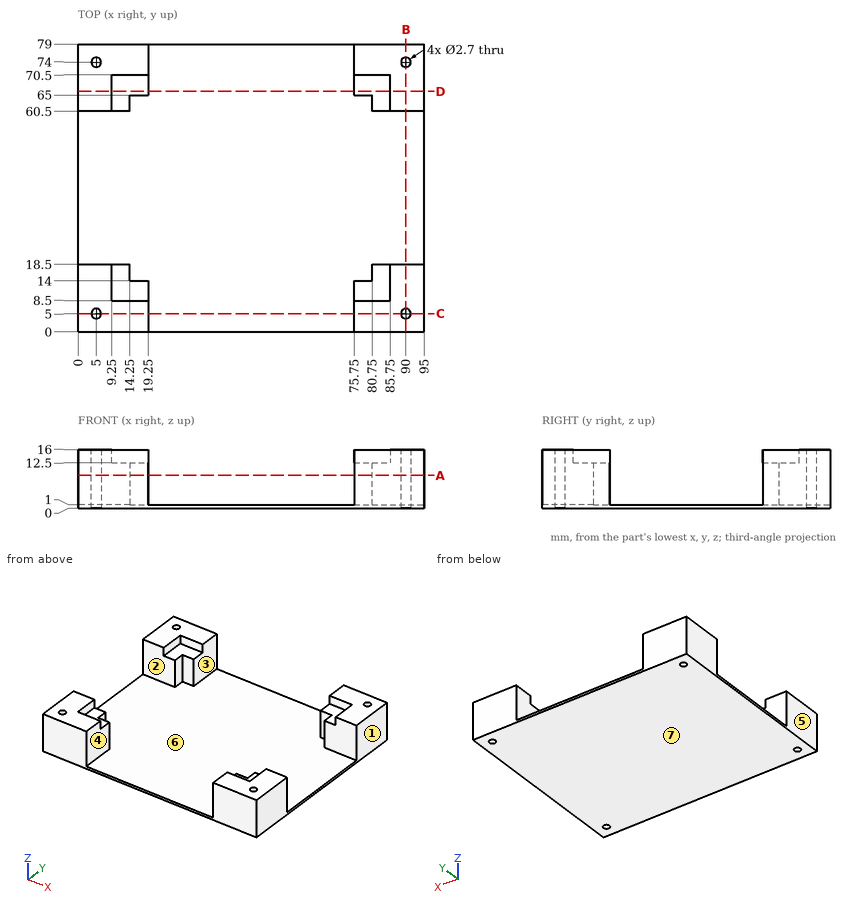
Can you work these out from the drawing? Everything is in mm from the part's minimum corner. A direction names the side the tool comes from. Round coordinates to 2 decimals unless told otherwise and drop trailing zeros. Write each loop counter-clockwise with the first axis right and the second up, starting at its lowest first coordinate (ties: lowest second). Pieces come first, ordered by that corner, then holes.
1. For the marked faces 1, 2 and 3, which set-ups out of +Z, -Z, +X, -X, +Y, -Y let a thin tool reach every point of the face, with its end or its side?
2. If we mould it in two halves opening along X, with no side actions, what happens to the marked faces 4, 5, 6 and 7? For each: released by +X, released by -X, zero draft, split by the parting line, or undercut.
3. I need wall thicknesses on L1, parallel to Y at x = 5, z = 5.25; L2, parallel to X at y = 74, z = 10.5; L3, parallel to Y at x = 79, z = 15.75. Which ranges of each line are inside material? Lowest first, please.
4. Suppose I cut it at D-D (y = 66). List the corners of the cut face in (x, z) for me.
5. Suppose I cut it at C-C (y = 5). List the corners of the cut face in (x, z) for me.
6. Will these pins go through, and if not, where does the flat tip stop? pin 1 Ø12 at (x, y) = (24.5, 26) entering from +Z; pin 2 Ø5 at (x, y) = (13.5, 11.5) entering from +Z; pin 3 Ø4 at (x, y) = (39.5, 60) entering from -Z.
7. Suppose I cut it at B-B (x = 90). List the corners of the cut face in (y, z) for me, and give its area (3 significant figures).
8. Suppose I cut it at A-A (z = 9). List the corners of the cut face in (x, y) for me, and give its area (3 significant figures).
Answer sheet:
1. face 1: +Z, -Z, +X, +Y, -Y
1. face 2: +Z, +X, -X
1. face 3: +Z, +Y, -Y
2. face 4: undercut
2. face 5: released by -X
2. face 6: undercut
2. face 7: zero draft
3. L1: y = 0 to 3.65, 6.35 to 18.5, 60.5 to 72.65, 75.35 to 79
3. L2: x = 0 to 3.65, 6.35 to 19.25, 75.75 to 88.65, 91.35 to 95
3. L3: y = 0 to 8.5, 70.5 to 79
4. outline: (0, 0) - (95, 0) - (95, 16) - (85.75, 16) - (85.75, 12.5) - (75.75, 12.5) - (75.75, 1) - (19.25, 1) - (19.25, 12.5) - (9.25, 12.5) - (9.25, 16) - (0, 16) - close
5. outline: (0, 0) - (3.65, 0) - (3.65, 16) - (0, 16) - close; (6.35, 0) - (88.65, 0) - (88.65, 16) - (75.75, 16) - (75.75, 1) - (19.25, 1) - (19.25, 16) - (6.35, 16) - close; (91.35, 0) - (95, 0) - (95, 16) - (91.35, 16) - close
6. pin 1: stops at z = 1
6. pin 2: stops at z = 12.5
6. pin 3: stops at z = 0
7. outline: (0, 0) - (3.65, 0) - (3.65, 16) - (0, 16) - close; (6.35, 0) - (72.65, 0) - (72.65, 16) - (60.5, 16) - (60.5, 1) - (18.5, 1) - (18.5, 16) - (6.35, 16) - close; (75.35, 0) - (79, 0) - (79, 16) - (75.35, 16) - close
7. area: 548 mm2
8. outline: (0, 0) - (19.25, 0) - (19.25, 14) - (14.25, 14) - (14.25, 18.5) - (0, 18.5) - close; (0, 60.5) - (14.25, 60.5) - (14.25, 65) - (19.25, 65) - (19.25, 79) - (0, 79) - close; (75.75, 0) - (95, 0) - (95, 18.5) - (80.75, 18.5) - (80.75, 14) - (75.75, 14) - close; (75.75, 65) - (80.75, 65) - (80.75, 60.5) - (95, 60.5) - (95, 79) - (75.75, 79) - close; hole circle Ø2.7 at (5, 5); hole circle Ø2.7 at (5, 74); hole circle Ø2.7 at (90, 5); hole circle Ø2.7 at (90, 74)
8. area: 1,310 mm2
